Part model, mm, in its own coordinate system. A direction names the side the tool comes from. Round coordinates to 2 decimals unless told otherwise and drop trailing zeros. Loops run counter-clockwise (first coordinate to the right, second up) from the corner with the lowest first, then second, coordinate; pieces in that order, holes last. Notation, with made-up numbers: M 32,-29 L 37,-29 A24 ccw 37,-6 Z; hole C 85.25,11 d3. An arc over 180 degrees is marked long. Put each result on its own line as item: value. Start each with the question number.
1) Slice it at B-B on x = -7. Give the cut face in (y, z), then the cut area to 3 significant figures.
2) Slice it at C-C on z = 10. State how many separate pieces and enclosed holes the cut face has, then the cut area to 3 significant figures.
3) Slice it at A-A on y = 3.5. Give the cut face in (x, z), then the cut area to 3 significant figures.
4) Which spindle directions (+Z, -Z, +X, -X, +Y, -Y) get a long thin tool onto all of the face, cutting with end or side? Do faces 5 (the cylindrical face through (-18.359, -36.797, 1.972)), 6 (the flat face through (16.5, 0, 8)), 7 (the cylindrical face through (-17, 36, 9)). Say none if no direction does.
5) Slice it at D-D on y = 18. Give the cut face in (x, z), then the cut area to 3 significant figures.
6) Pull direction X, two halves, no side cores. Call faces 1 (the flat face through (-16.5, 0, 8)), 2 (the flat face through (-19.5, 0, 2)), 3 (the flat face through (-1, 7, 7)), 4 (the flat face through (0, -38, 2)): +X half, -X half, draft (parallel to the pull), parting line (faces both ways), or undercut.
7) Probe line 1 along Y through (x, z) = (-2, 8.75); line 2 along X through (y, z) = (-7.5, 3); line 3 along Y through (x, z) = (1.5, 7.75). List the from-to ranges inside material, lowest first.
8) Drop flat-ended pins along their axis: pin 1 Ø0.7 at (x, y) = (-12.5, -19) entering from +Z; pin 2 Ø1.5 at (y, z) = (8, 5.5) entering from -X; pin 3 Ø0.9 at (y, z) = (8, 7) entering from +X. Give the stop position or say it passes through.
```python
from build123d import *

# Parameters (mm, degrees)
F1_DEPTH      = 2
F3_DEPTH      = 2
F5_W          = 12
F5_H          = 3
F6_DEPTH      = 8
F6_DEPTH_BACK = 2
F8_DEPTH      = 50
F10_DEPTH     = 50
F11_DEPTH     = 10


with BuildPart() as f1:
    # F0 (on Top) → F1 (new body)
    with BuildSketch(Plane.XY):
        with BuildLine():
            Line((-15.5, -38), (15.5, -38))
            ThreePointArc((15.5, -38), (18.3284271247, -36.8284271247), (19.5, -34))
            Line((19.5, -34), (19.5, 34))
            ThreePointArc((19.5, 34), (18.3284271247, 36.8284271247), (15.5, 38))
            Line((15.5, 38), (-15.5, 38))
            ThreePointArc((-15.5, 38), (-18.3284271247, 36.8284271247), (-19.5, 34))
            Line((-19.5, 34), (-19.5, -34))
            ThreePointArc((-19.5, -34), (-18.3284271247, -36.8284271247), (-15.5, -38))
        make_face()
    extrude(amount=F1_DEPTH)

    # F2 (on face) → F3 (join)
    with BuildSketch(Plane.XY.offset(2)):
        with BuildLine():
            Line((-19.5, 34), (-19.5, -34))
            ThreePointArc((-19.5, -34), (-18.3284271247, -36.8284271247), (-15.5, -38))
            Line((-15.5, -38), (15.5, -38))
            ThreePointArc((15.5, -38), (18.3284271247, -36.8284271247), (19.5, -34))
            Line((19.5, -34), (19.5, 34))
            ThreePointArc((19.5, 34), (18.3284271247, 36.8284271247), (15.5, 38))
            Line((15.5, 38), (-15.5, 38))
            ThreePointArc((-15.5, 38), (-18.3284271247, 36.8284271247), (-19.5, 34))
        make_face()
        with BuildLine():
            ThreePointArc((-15.5, -34.9999999106), (-16.207106718, -34.707106718), (-16.4999999106, -34))
            Line((-16.4999999106, -34), (-16.4999999106, 34))
            ThreePointArc((-16.4999999106, 34), (-16.207106718, 34.707106718), (-15.5, 34.9999999106))
            Line((-15.5, 34.9999999106), (15.5, 34.9999999106))
            ThreePointArc((15.5, 34.9999999106), (16.207106718, 34.707106718), (16.4999999106, 34))
            Line((16.4999999106, 34), (16.4999999106, -34))
            ThreePointArc((16.4999999106, -34), (16.207106718, -34.707106718), (15.5, -34.9999999106))
            Line((15.5, -34.9999999106), (-15.5, -34.9999999106))
        make_face(mode=Mode.SUBTRACT)
    extrude(amount=F3_DEPTH)

    # F5 (on face) → F6 (join, two sides)
    with BuildSketch(Plane.XY.offset(4)) as f6_sk:
        with Locations((-7, -18.4999999106)):
            Rectangle(F5_W, F5_H)
        with Locations((-7, 7.5000000894)):
            Rectangle(F5_W, F5_H)
        with Locations((7, 18.4999999106)):
            Rectangle(F5_W, F5_H)
        with Locations((7, -7.5000000894)):
            Rectangle(F5_W, F5_H)
    extrude(amount=F6_DEPTH)
    extrude(f6_sk.sketch, amount=-F6_DEPTH_BACK)

    # F7 (on face) → F8 (cut)
    with BuildSketch(Plane.XZ.offset(19.9999999106)):
        with BuildLine():
            Line((-1.9, 12), (-12.1, 12))
            ThreePointArc((-12.1, 12), (-7, 6.9), (-1.9, 12))
        make_face()
    extrude(amount=-F8_DEPTH, mode=Mode.SUBTRACT)

    # F9 (on face) → F10 (cut)
    with BuildSketch(Plane.XZ.offset(9.0000000894)):
        with BuildLine():
            Line((12.1, 12), (1.9, 12))
            ThreePointArc((1.9, 12), (7, 6.9), (12.1, 12))
        make_face()
    extrude(amount=-F10_DEPTH, mode=Mode.SUBTRACT)

    # F4 (on face) → F11 (join)
    with BuildSketch(Plane.XY.offset(4)):
        with BuildLine():
            Line((-18, 34), (-18, -34))
            ThreePointArc((-18, -34), (-17.267766953, -35.767766953), (-15.5, -36.5))
            Line((-15.5, -36.5), (15.5, -36.5))
            ThreePointArc((15.5, -36.5), (17.267766953, -35.767766953), (18, -34))
            Line((18, -34), (18, 34))
            ThreePointArc((18, 34), (17.267766953, 35.767766953), (15.5, 36.5))
            Line((15.5, 36.5), (-15.5, 36.5))
            ThreePointArc((-15.5, 36.5), (-17.267766953, 35.767766953), (-18, 34))
        make_face()
        with BuildLine():
            ThreePointArc((-15.5, -34.9999999106), (-16.207106718, -34.707106718), (-16.4999999106, -34))
            Line((-16.4999999106, -34), (-16.4999999106, 34))
            ThreePointArc((-16.4999999106, 34), (-16.207106718, 34.707106718), (-15.5, 34.9999999106))
            Line((-15.5, 34.9999999106), (15.5, 34.9999999106))
            ThreePointArc((15.5, 34.9999999106), (16.207106718, 34.707106718), (16.4999999106, 34))
            Line((16.4999999106, 34), (16.4999999106, -34))
            ThreePointArc((16.4999999106, -34), (16.207106718, -34.707106718), (15.5, -34.9999999106))
            Line((15.5, -34.9999999106), (-15.5, -34.9999999106))
        make_face(mode=Mode.SUBTRACT)
    extrude(amount=F11_DEPTH)


solid = f1.part
```
Recorded:
1. outline: M -38,0 L 38,0 L 38,4 L 36.5,4 L 36.5,14 L 35,14 L 35,2 L 9,2 L 9,6.9 L 6,6.9 L 6,2 L -17,2 L -17,6.9 L -20,6.9 L -20,2 L -35,2 L -35,14 L -36.5,14 L -36.5,4 L -38,4 Z
1. area: 223 mm2
2. separate pieces: 9
2. enclosed holes: 1
2. area: 345 mm2
3. outline: M -19.5,0 L 19.5,0 L 19.5,4 L 18,4 L 18,14 L 16.5,14 L 16.5,2 L -16.5,2 L -16.5,14 L -18,14 L -18,4 L -19.5,4 Z
3. area: 120 mm2
4. face 5: +Z, -Z, -X, -Y
4. face 6: +Z
4. face 7: +Z, -X, +Y
5. outline: M -19.5,0 L 19.5,0 L 19.5,4 L 18,4 L 18,14 L 16.5,14 L 16.5,2 L 13,2 L 13,12 L 12.1,12 A5.1 cw 1.9,12 L 1,12 L 1,2 L -16.5,2 L -16.5,14 L -18,14 L -18,4 L -19.5,4 Z
5. area: 199 mm2
6. face 1: undercut
6. face 2: -X half
6. face 3: undercut
6. face 4: draft
7. line 1: y = -36.5 to -35, -20 to -17, 6 to 9, 35 to 36.5
7. line 2: x = -19.5 to -16.5, 1 to 13, 16.5 to 19.5
7. line 3: y = -36.5 to -35, -9 to -6, 17 to 20, 35 to 36.5
8. pin 1: stops at z = 12
8. pin 2: stops at x = -18
8. pin 3: stops at x = 18
